Autodesk Inventor part; units mm, degrees
ref_plane "YZ Plane" through (0, 0, 0) normal (1, 0, 0) x (0, 1, 0)
ref_plane "XZ Plane" through (0, 0, 0) normal (0, 1, 0) x (-1, 0, 0)
ref_plane "XY Plane" through (0, 0, 0) normal (0, 0, 1) x (1, 0, 0)
sketch "Sketch1" plane through (0, 0, 0) normal (0, 0, 1) x (1, 0, 0)
  point P0 (0, 0)
sketch "Sketch2" plane through (0, 0, 0) normal (0, 0, 1) x (1, 0, 0)
  line L0 (0, 4.445) -> (0, -4.445)
  line L1 (-4.445, 0) -> (4.445, 0)
  circle A0 centre (0, 0) radius 3.175
  dimension "d0" = 6.35
extrude "Extrusion1" add sketch "Sketch2" along normal blind 109.22
sketch "Sketch3" plane through (0, 0, 0) normal (1, 0, 0) x (0, 1, 0)
  line L0 (0, 29.718) -> (0, -4.953)
  line L1 (-4.445, 0) -> (4.445, 0)
  line L2 (-3.175, 0) -> (3.175, 0)
  line L3 (-3.175, 0) -> (-0.7874, 0)
  line L4 (-0.7874, 0) -> (-0.7874, 24.765)
  line L5 (-0.7874, 24.765) -> (-3.175, 24.765)
  line L6 (-3.175, 24.765) -> (-3.175, 0)
  line L7 (-0.7874, 24.765) -> (-0.2794, 24.765)
  line L8 (-0.2794, 24.765) -> (-0.2794, 23.241)
  line L9 (-0.2794, 23.241) -> (-0.7874, 23.241)
  line L10 (-0.7874, 23.241) -> (-0.7874, 24.765)
  point P0 (0, 0)
  dimension "d3" = 24.765
  dimension "d4" = 0.508
  dimension "d5" = 1.524
  dimension "d6" = 3.9624
extrude "Extrusion2" cut sketch "Sketch3" along normal mid plane 25.4
sketch "Sketch4" plane through (0, -0.7874, -0.635) normal (0, 1, 0) x (-1, 0, 0)
  line L0 (-3.0758, 0.635) -> (3.0758, 0.635)
  line L1 (0, -21.209) -> (0, 131.699)
  line L2 (3.1627, 25.4) -> (-3.1627, 25.4)
  point P0 (0, 0.635)
  point P1 (0, 9.398)
  point P2 (3.1627, 25.4)
  point P3 (-3.1627, 25.4)
  point P4 (0, 20.398)
  dimension "d13" = 16.002
  dimension "d14" = 11
hole "Hole1" at (0, -0.7874, 8.763) at (0, -0.7874, 19.763) direction (0, 1, 0) diameter 1.5748 end through all
chamfer "Chamfer1" distance 0.762 angle 45 1 edges at (-3.175, 0, 109.22)
sketch "Sketch5" plane through (0, 0, 0) normal (1, 0, 0) x (0, 1, 0)
  line L0 (3.175, 0) -> (3.175, 108.458)
  line L1 (-1.5799, 0) -> (3.9675, 0)
  line L2 (3.175, 0) -> (3.175, 7.2044)
  line L3 (3.175, 7.2044) -> (1.2446, 0)
  line L4 (-0.7874, 0) -> (3.175, 0)
  line L5 (1.2446, 0) -> (3.175, 0)
  line L6 (-0.7874, 0) -> (-0.7874, 23.241)
  point P0 (0, 0)
  dimension "d22" = 1.9304
  dimension "d26" = 2.032
  dimension "d27" = 15
extrude "Extrusion3" cut sketch "Sketch5" along normal mid plane 25.4
properties part number "J007626" material "ALUMINUM, 6061-T651"
CAD build for the part. Positions are in the model's coordinates, mm. A direction names the side the tool comes from. Round coordinates to 2 decimals unless told otherwise and drop trailing zeros. Loops run counter-clockwise (first coordinate to the right, second up) from the corner with the lowest first, then second, coordinate; pieces in that order, holes last.
(1) Wall check: line 1 along Z through (x, y) = (0, 0.4); line 2 along Z through (x, y) = (-0.5, 1); line 3 along Y through (x, z) = (-0.25, 21.5). Give the ranges that are in metal, low to high.
(2) Which spindle directions (+Z, -Z, +X, -X, +Y, -Y) get a long thin tool onto all of the face, cutting with end or side? Do faces 1 (the flat face through (-0.04, 2.01, 2.85)), 2 (the flat face through (0, -0.787, 11)). Say none if no direction does.
(3) Two-plate mould, pull along Z, no slides. Class faces 3 (the flat face through (0, -1, 24.765)), 4 (the flat face through (0, 0, 109.22)), 5 (the cylindrical face through (-0.69, 3.1, 65.52)), 6 (the flat face through (0, 0, 0)): +Z half, -Z half, draft (parallel to the pull), parting line (faces both ways), or undercut.
(4) Cut at A-A (z = 96.5). Give the cut face in (x, y) (3 decimals), plus the area to 3 significant figures.
(5) Drop flat-ended pins along their axis: pin 1 (0.8 mm diameter, centred on x = -1, z = 24, fed in from -Y); pin 2 (1 mm diameter, centred on x = 0, y = 0, fed in from -Z); pin 3 (1 mm diameter, centred on x = 1, z = 40.5, fed in from -Y); pin 4 (2.5 mm diameter, centred on x = 0.5, y = -2.5, fed in from -Z) (3 decimals). Give the stop position or say it passes through.
Findings below:
1. line 1: z = 0 to 7.98, 9.55 to 18.98, 20.55 to 109.22
1. line 2: z = 0 to 8.15, 9.37 to 19.15, 20.37 to 109.22
1. line 3: y = -0.79 to 3.17
2. face 1: -Z, +X, -X, +Y
2. face 2: -Z, +X, -X, -Y
3. face 3: undercut
3. face 4: +Z half
3. face 5: draft
3. face 6: -Z half
4. outline: circle Ø6.35 at (0, 0)
4. area: 31.7 mm2
5. pin 1: stops at y = -0.28
5. pin 2: stops at z = 0
5. pin 3: stops at y = -3.14
5. pin 4: stops at z = 24.765
